from build123d import *

# Parameters (mm, degrees)
F0_R     = 12.7
F1_DEPTH = 280
F2_R     = 15.875
F3_DEPTH = 50
F4_R     = 11.684
F5_DEPTH = 270.476


with BuildPart() as f1:
    # F0 (on Top) → F1 (new body)
    with BuildSketch(Plane.XY):
        Circle(F0_R)
    extrude(amount=F1_DEPTH)

    # F2 (on Right) → F3 (cut, symmetric)
    with BuildSketch(Plane.YZ):
        Circle(F2_R)
    extrude(amount=F3_DEPTH, both=True, mode=Mode.SUBTRACT)

    # F4 (on face) → F5 (cut, through all)
    with BuildSketch(Plane.XY.offset(280)):
        Circle(F4_R)
    extrude(amount=-F5_DEPTH, mode=Mode.SUBTRACT)


solid = f1.part
Verification items for the finished model (mm, model axes). Coordinates: 2 decimals unless noted, no trailing zeros. Write each loop counter-clockwise with the first axis right and the second up, starting at its lowest first coordinate (ties: lowest second). Pieces come first, ordered by that corner, then holes. Notation, with made-up numbers: (89.5, 82) - (96.5, 82) arc R16 ccw to (96.5, 101) - close; hole circle Ø6 at (0.25, 39). An arc over 180 degrees is marked (long way). Answer as a JSON object with one key per item and string values.
(1) Cross-section at A-A on x = 0. Record the cut outline in (y, z) (3 decimals).
Report:
{"outline": "(-12.7, 9.525) arc R15.875 cw to (-11.684, 10.747) - (-11.684, 280) - (-12.7, 280) - close; (11.684, 10.747) arc R15.875 cw to (12.7, 9.525) - (12.7, 280) - (11.684, 280) - close"}
(2) Gauge pin test, flat ends, axial feed: pin 1 Ø8 at (y, z) = (-5, 105.5) entering from -X; pin 2 Ø5 at (y, z) = (4.5, 218.5) entering from -X; pin 3 Ø6 at (y, z) = (-8.5, 140) entering from -X. Record the tip position at first contact, or that the pin passes through.
Report:
{"pin 1": "x = -12.66", "pin 2": "x = -12.54", "pin 3": "x = -11.45"}
(3) Mould release check, pull along Y, two halves, no side actions. Record for faces 1 (the flat face through (8.4, -8.4, 280)), 2 (the cylindrical face through (-2.75, -12.4, 142.87)), 3 (the cylindrical face through (-8.43, 8.35, 13.5)): pulls with the +Y half, pulls with the -Y half, needs draft (parallel to the pull), parting line crosses it, or undercut.
Report:
{"face 1": "needs draft", "face 2": "parting line crosses it", "face 3": "undercut"}
(4) Cross-section at B-B on y = 0. Record the cut outline in (x, z) (3 decimals).
Report:
{"outline": "(-12.7, 15.875) - (-11.684, 15.875) - (-11.684, 280) - (-12.7, 280) - close; (11.684, 15.875) - (12.7, 15.875) - (12.7, 280) - (11.684, 280) - close"}
(5) Cross-section at C-C on z = 101. Record the cut outline in (x, y), plus the area to 3 significant figures.
Report:
{"outline": "circle Ø25.4 at (0, 0); hole circle Ø23.37 at (0, 0)", "area": "77.8 mm^2"}
(6) Thickness scan on line 1 along Y through (x, z) = (0, 133.5); line 2 along Y through (x, z) = (3, 28.5). Record the ranges inside material, lowest first.
Report:
{"line 1": "-12.7 to -11.68, 11.68 to 12.7", "line 2": "-12.34 to -11.29, 11.29 to 12.34"}
